Source: CAD feature listing. Evaluate the final solid. Frame: model axes, mm. A direction names the side the tool comes from. Coordinates: 2 decimals unless noted, no trailing zeros. Write each loop counter-clockwise with the first axis right and the second up, starting at its lowest first coordinate (ties: lowest second). Pieces come first, ordered by that corner, then holes. Notation, with made-up numbers: M 64,34.5 L 114,34.5 A24 cw 114,62.5 Z; hole C 78.5,68 d10. An arc over 180 degrees is marked long. One line per item, written item: value. Start each with the question number.
Item 1: Set-up query: faces 1 (the cylindrical face through (-0.1, 92.9, 4.9)), 2 (the cylindrical face through (0, -1.9, 4.9)). Return all of +Z, -Z, +X, -X, +Y, -Y with unobstructed straight access to the full face (end or side cutting, diameter ignored); none if empty.
Item 2: Ray query, L1, parallel to X at y = 21.5, z = 9; L2, parallel to Y at x = 1.1, z = 6; L3, parallel to Y at x = -0.25, z = 8. Return the intervals inside material, ascending. Write a range as from..to.
Item 3: Cut plane A-A, the plane y = 19. Output: boundary loops of the cut face in (x, z), then the cut area to 3 significant figures.
Item 4: Mould query, pull axis Y, two halves, no side actions, for faces 3 (the cylindrical face through (0.1, -2.9, 4.9)), 4 (the flat face through (1.9, 46, 5)), 5 (the flat face through (2.9, 46, 5)). Classes: released by +Y, released by -Y, zero draft, split by the parting line, or undercut.
Item 5: Cut plane C-C, the plane z = 6.5. Output: boundary loops of the cut face in (x, y).
Item 6: Cut plane B-B, the plane x = 0. Output: boundary loops of the cut face in (y, z), then the cut area to 3 significant figures.
```python
from build123d import *

# Parameters (mm, degrees)
SURFACE_EXTRUDE1_1_DEPTH = 10
THICKEN1_T1              = 1


with BuildPart() as body_1:
    # Surface-Extrude1: a surface, the sketch's curves swept straight by 10 mm
    with BuildLine(Plane.XY, mode=Mode.PRIVATE) as surface_extrude1_1_path:
        Line((-1.9, 0), (-1.9, 90))
        ThreePointArc((-1.9, 90), (0, 91.9), (1.9, 90))
        Line((1.9, 90), (1.9, 0))
        ThreePointArc((1.9, 0), (0, -1.9), (-1.9, 0))
    surface_extrude1_1 = Shell.extrude(surface_extrude1_1_path.wire(), (0 * SURFACE_EXTRUDE1_1_DEPTH, 0 * SURFACE_EXTRUDE1_1_DEPTH, 1 * SURFACE_EXTRUDE1_1_DEPTH))
    add(Solid.thicken(surface_extrude1_1, THICKEN1_T1))


solid = body_1.part
```
From the geometry:
1. face 1: +Z, -Z, +Y
1. face 2: +Z, -Z
2. L1: x = -2.9..-1.9, 1.9..2.9
2. L2: y = -2.68..-1.55, 91.55..92.68
2. L3: y = -2.89..-1.88, 91.88..92.89
3. outline: M -2.9,0 L -1.9,0 L -1.9,10 L -2.9,10 Z; M 1.9,0 L 2.9,0 L 2.9,10 L 1.9,10 Z
3. area: 20.0 mm²
4. face 3: released by -Y
4. face 4: undercut
4. face 5: zero draft
5. outline: M -2.9,0 A2.9 ccw 2.9,0 L 2.9,90 A2.9 ccw -2.9,90 Z; hole M -1.9,0 A1.9 ccw 1.9,0 L 1.9,90 A1.9 ccw -1.9,90 Z
6. outline: M -2.9,0 L -1.9,0 L -1.9,10 L -2.9,10 Z; M 91.9,0 L 92.9,0 L 92.9,10 L 91.9,10 Z
6. area: 20.0 mm²
